Geometry check sheet. Reference: the model listing, model coordinates, mm. Coordinates: 2 decimals unless noted, no trailing zeros. Order: outer loops, then holes, each group sorted by start corner. A loop starts at its lowest first (then second) coordinate and runs counter-clockwise, first axis right, second up. Notation, with made-up numbers: (63.25, 80) - (97.25, 80) arc R23 cw to (97.25, 88) - close; hole circle Ø5 at (62, 28.5). An arc over 180 degrees is marked (long way). Put each result on its own line as item: value.
from build123d import *

# Parameters (mm, degrees)
BOSS_EXTRUDE1_DEPTH        = 1.6002
F_2_7_2_7_DIAMETER_HOLE1_D = 2.75


with BuildPart() as part:
    # Sketch1 → Boss-Extrude1 (new body)
    with BuildSketch(Plane(origin=(0, 0, 0), x_dir=(1, 0, 0), z_dir=(0, 1, 0))):
        with BuildLine():
            Line((3, 0), (53, 0))
            ThreePointArc((53, 0), (55.121320344, 0.878679656), (56, 3))
            Line((56, 3), (56, 62))
            ThreePointArc((56, 62), (55.121320344, 64.121320344), (53, 65))
            Line((53, 65), (3, 65))
            ThreePointArc((3, 65), (0.878679656, 64.121320344), (0, 62))
            Line((0, 62), (0, 3))
            ThreePointArc((0, 3), (0.878679656, 0.878679656), (3, 0))
        make_face()
    extrude(amount=BOSS_EXTRUDE1_DEPTH)

    # Ø2.7 (2.7) Diameter Hole1 (through all)
    with Locations(Plane(origin=(0, 1.6002, 0), x_dir=(1, 0, 0), z_dir=(0, 1, 0))):
        with Locations((3.5, 61.5), (3.5, 3.5), (52.5, 61.5), (52.5, 3.5)):
            Hole(F_2_7_2_7_DIAMETER_HOLE1_D / 2)


solid = part.part
Q1. Thickness scan on L1, parallel to Z at x = 52.5, y = 0.6 (3 decimals); L2, parallel to X at y = 0.9, z = -61.5 (3 decimals); L3, parallel to Z at x = 54.5, y = 1.5. Record the ranges inside material, lowest first. Write a range as [from, to].
Answer block:
L1: z = [-65, -62.875], [-60.125, -4.875], [-2.125, 0]
L2: x = [0, 2.125], [4.875, 51.125], [53.875, 56]
L3: z = [-64.6, -0.4]
Q2. Section check A-A on x = 52. Record the boundary of the cut face in (y, z), then the cut area to 3 significant figures.
Answer block:
outline: (0, -65) - (1.6, -65) - (1.6, -62.78) - (0, -62.78) - close; (0, -60.22) - (1.6, -60.22) - (1.6, -4.78) - (0, -4.78) - close; (0, -2.22) - (1.6, -2.22) - (1.6, 0) - (0, 0) - close
area: 95.8 mm^2
Q3. Draft check along X on faces 1 (the flat face through (0, 1, -33)), 2 (the cylindrical face through (55.14, 0.79, -64.1)), 3 (the flat face through (28, 1.6, -33)), 4 (the cylindrical face through (53.874, 0.789, -3.56)). Enter one of: pulls with the +X half, pulls with the -X half, needs draft (parallel to the pull), parting line crosses it, or undercut.
Answer block:
face 1: pulls with the -X half
face 2: pulls with the +X half
face 3: needs draft
face 4: undercut
